Model file for the job. Use its own axes, mm. A direction names the side the tool comes from. Give positions to 0.01 mm unless a question says otherwise; leave off trailing zeros.
```python
from build123d import *

# Parameters (mm, degrees)
SKETCH_1_R      = 25
EXTRUDE_1_DEPTH = 1
FILLET_1_R      = 1.6
EXTRUDE_START   = 5
EXTRUDE_3_DEPTH = 5
CHAMFER_3_SIZE  = 0.2


with BuildPart() as part:
    # 草图1 → 凸台-拉伸1 (new body)
    with BuildSketch(Plane.XY):
        Circle(SKETCH_1_R)
        with BuildLine():
            Line((-5.908846518, 1.041889066), (-7.878462024, 1.389185421))
            ThreePointArc((-7.878462024, 1.389185421), (-7.72740661, 2.070552361), (-7.517540966, 2.736161147))
            Line((-7.517540966, 2.736161147), (-5.638155725, 2.05212086))
            ThreePointArc((-5.638155725, 2.05212086), (-5.795554958, 1.552914271), (-5.908846518, 1.041889066))
        make_face(mode=Mode.SUBTRACT)
        with BuildLine():
            Line((-2.5, 1.658312395), (2.5, 1.658312395))
            ThreePointArc((2.5, 1.658312395), (0, -3), (-2.5, 1.658312395))
        make_face(mode=Mode.SUBTRACT)
        with BuildLine():
            ThreePointArc((-12.124355653, -7), (-7, -12.124355653), (0, -14))
            Line((0, -14), (0, -21))
            ThreePointArc((0, -21), (-10.5, -18.186533479), (-18.186533479, -10.5))
            Line((-18.186533479, -10.5), (-12.124355653, -7))
        make_face(mode=Mode.SUBTRACT)
        with BuildLine():
            ThreePointArc((0, 14), (-7, 12.124355653), (-12.124355653, 7))
            Line((-12.124355653, 7), (-18.186533479, 10.5))
            ThreePointArc((-18.186533479, 10.5), (-10.5, 18.186533479), (0, 21))
            Line((0, 21), (0, 14))
        make_face(mode=Mode.SUBTRACT)
        with BuildLine():
            ThreePointArc((18.186533479, 10.5), (21, 0), (18.186533479, -10.5))
            Line((18.186533479, -10.5), (12.124355653, -7))
            ThreePointArc((12.124355653, -7), (14, 0), (12.124355653, 7))
            Line((12.124355653, 7), (18.186533479, 10.5))
        make_face(mode=Mode.SUBTRACT)
    extrude(amount=-EXTRUDE_1_DEPTH)

    # 圆角1
    fillet_1_edges = [part.edges().sort_by_distance(p)[0] for p in [
        (-18.186533479, -10.5, -0.5),
        (0, -21, -0.5),
        (0, -14, -0.5),
        (-12.124355653, -7, -0.5),
        (18.186533479, -10.5, -0.5),
        (18.186533479, 10.5, -0.5),
        (12.124355653, 7, -0.5),
        (12.124355653, -7, -0.5),
        (-18.186533479, 10.5, -0.5),
        (-12.124355653, 7, -0.5),
        (0, 14, -0.5),
        (0, 21, -0.5),
    ]]
    fillet(fillet_1_edges, radius=FILLET_1_R)

    # 草图1<5> → 凸台-拉伸3 (add)
    with BuildSketch(Plane.XY.offset(EXTRUDE_START)):
        with BuildLine():
            ThreePointArc((-1.5, 2.598076211), (-2.054455891, 2.186140662), (-2.5, 1.658312395))
            Line((-2.5, 1.658312395), (2.5, 1.658312395))
            ThreePointArc((2.5, 1.658312395), (2.054455891, 2.186140662), (1.5, 2.598076211))
            Line((1.5, 2.598076211), (3, 5.196152423))
            ThreePointArc((3, 5.196152423), (0, 6), (-3, 5.196152423))
            Line((-3, 5.196152423), (-1.5, 2.598076211))
        make_face()
        with BuildLine():
            ThreePointArc((-1.5, -2.598076211), (-2.598076211, -1.5), (-3, 0))
            Line((-3, 0), (-6, 0))
            ThreePointArc((-6, 0), (-5.196152423, -3), (-3, -5.196152423))
            Line((-3, -5.196152423), (-1.5, -2.598076211))
        make_face()
        with BuildLine():
            Line((6, 0), (3, 0))
            ThreePointArc((3, 0), (2.598076211, -1.5), (1.5, -2.598076211))
            Line((1.5, -2.598076211), (3, -5.196152423))
            ThreePointArc((3, -5.196152423), (5.196152423, -3), (6, 0))
        make_face()
    extrude(amount=-EXTRUDE_3_DEPTH)

    # 倒角3
    chamfer_3_edges = [part.edges().sort_by_distance(p)[0] for p in [
        (18.021198676, 9.808386563, -1),
        (12.716572017, 6.866149549, -1),
        (12.716572017, -6.866149549, -1),
        (-17.504911272, 10.702622579, -1),
        (-12.304545944, 7.579799641, -1),
        (-0.412026073, 14.44594919, -1),
        (-0.516287404, 20.511009142, -1),
        (0, 1.658312395, -1),
        (-7.72740661, 2.070552361, -1),
        (-2.25, 3.897114317, 5),
        (0, 1.658312395, 5),
        (2.054455891, 2.186140662, 5),
        (2.25, 3.897114317, 5),
        (0, 6, 5),
        (-2.054455891, 2.186140662, 5),
        (-2.25, -3.897114317, 5),
        (-2.598076211, -1.5, 5),
        (-4.5, 0, 5),
        (-5.196152423, -3, 5),
        (4.5, 0, 5),
        (2.598076211, -1.5, 5),
        (2.25, -3.897114317, 5),
        (5.196152423, -3, 5),
        (-6.577848346, 2.394141003, -1),
        (-5.795554958, 1.552914271, -1),
        (-6.893654271, 1.215537244, -1),
        (-25, 0, -1),
        (-10.5, -18.186533479, -1),
        (-15.091202728, -8.712909958, -1),
        (-7, -12.124355653, -1),
        (0, -17.425819915, -1),
        (21, 0, -1),
        (15.091202728, -8.712909958, -1),
        (15.091202728, 8.712909958, -1),
        (14, 0, -1),
        (-15.091202728, 8.712909958, -1),
        (-10.5, 18.186533479, -1),
        (-7, 12.124355653, -1),
        (0, 17.425819915, -1),
        (-17.504911272, -10.702622579, -1),
        (0, -3, -1),
        (-12.304545944, -7.579799641, -1),
        (-0.412026073, -14.44594919, -1),
        (-0.516287404, -20.511009142, -1),
        (18.021198676, -9.808386563, -1),
    ]]
    chamfer(chamfer_3_edges, length=CHAMFER_3_SIZE)


solid = part.part
```
1. Which spindle directions (+Z, -Z, +X, -X, +Y, -Y) get a long thin tool onto all of the face, cutting with end or side? Do faces 4 (the cylindrical face through (5.174, -3.038, 2.434)), 5 (the cylindrical face through (-0.423, -14.434, -0.406)). Say none if no direction does.
Calculated:
face 4: +Z, +X, -Y
face 5: +Z, -Z
2. Slice it at A-A, the plane x = -15.5. State how many separate pieces and enclosed holes the cut face has, and give its area (3 significant figures).
Calculated:
separate pieces: 3
enclosed holes: 0
area: 28.6 mm2
3. Pin check, flat tips, straight feed: P1, Ø3.5, axis at x = 5, z = 2.5, coming from the +Y side; P2, Ø2, axis at y = -2, z = 1.5, coming from the +X side; P3, Ø5, axis at x = -18.5, y = 18, coming from the +Z side. Stop position of each tip, or through.
Calculated:
P1: stops at y = 0
P2: stops at x = 5.92
P3: stops at z = 0
4. Pull direction X, two halves, no side cores. Call faces 1 (the flat face through (2.24, 3.88, 2.43)), 2 (the flat face through (-2.26, -3.915, 2.434)), 3 (the flat face through (-4, 0, 2)): +X half, -X half, draft (parallel to the pull), parting line (faces both ways), or undercut.
Calculated:
face 1: +X half
face 2: undercut
face 3: draft
5. Probe probe 1 along Z at (x, y) = (-19, -7); probe 2 along Z at (x, y) = (-14, 8); probe 3 along Y at (x, z) = (4, 2). List the from-to ranges inside material, lowest first.
Calculated:
probe 1: z = -1 to 0
probe 2: z = -0.87 to 0
probe 3: y = -4.47 to 0
